Study the drawing (mm; zero at the part's minimum x, y, z) and answer. A direction names the side the tool comes from. Coordinates: 2 decimals unless noted, no trailing zeros. Order: outer loops, then holes, each group sorted by start corner. A loop starts at its lowest first (then second) coordinate and runs counter-clockwise, first axis right, second up. Notation, with made-up numbers: M 27.5,-13.75 L 81.5,-13.75 A16 cw 81.5,6.25 Z; hole C 13,-0.5 d10. An arc over 180 degrees is marked long. Use a Markdown table: item, result. Add a question column.
1) Find section C-C on z = 7.5. Write down the section's boundary in (x, y).
2) Find section D-D on y = 3.25. Write down the section's boundary in (x, z).
3) For the marked faces 1, 2 and 3, determine the directions among +Z, -Z, +X, -X, +Y, -Y from which every point of the face is accessible in a straight line to the end or side of a thin tool.
4) Each of these flat-tipped pins is pushed along its axis until it touches: pin 1 Ø1.5 at (y, z) = (15, 16) entering from +X; pin 2 Ø1 at (x, z) = (5.5, 5) entering from -Y; pin 3 Ø3 at (x, z) = (5, 15.5) entering from -Y; pin 4 Ø1 at (x, z) = (3, 9.5) entering from +Y. Where does it stop, or does it pass through?
5) Find section A-A on y = 10.16. Write down the section's boundary in (x, z), plus the area to 3 significant figures.
6) Find the intervals of material crossed by probe 1 along Z at (x, y) = (17.25, 16.25); probe 2 along Y at (x, z) = (5, 22); probe 3 along Y at (x, z) = (8.75, 7.5), in increasing order. Write a range as [from, to].
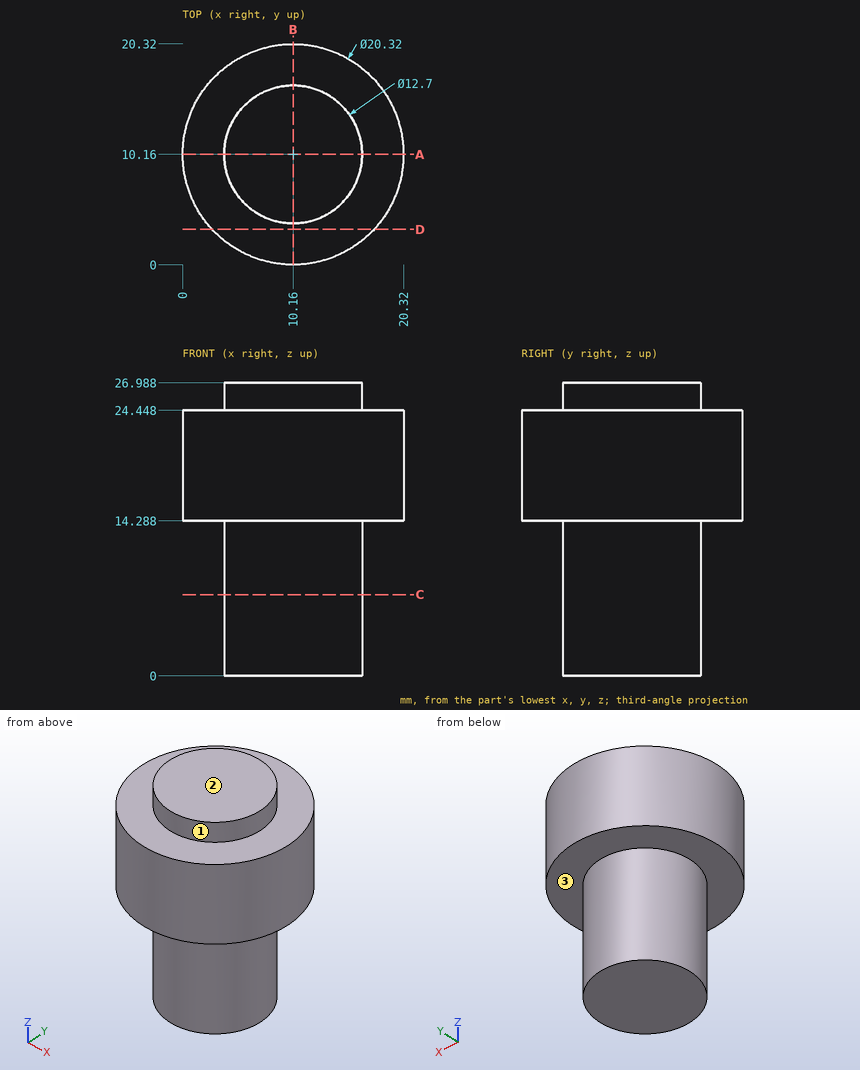
Check result:
| question | item | result |
|---|---|---|
| 1 | outline | C 10.16,10.16 d12.7 |
| 2 | outline | M 2.71,14.29 L 17.61,14.29 L 17.61,24.45 L 2.71,24.45 Z |
| 3 | face 1 | +Z |
| 3 | face 2 | +Z, +X, -X, +Y, -Y |
| 3 | face 3 | -Z |
| 4 | pin 1 | stops at x = 19.46 |
| 4 | pin 2 | stops at y = 5.36 |
| 4 | pin 3 | stops at y = 0.68 |
| 4 | pin 4 | passes through |
| 5 | outline | M 0,14.29 L 3.81,14.29 L 3.81,0 L 16.51,0 L 16.51,14.29 L 20.32,14.29 L 20.32,24.45 L 16.51,24.45 L 16.51,26.99 L 3.81,26.99 L 3.81,24.45 L 0,24.45 Z |
| 5 | area | 420 mm2 |
| 6 | probe 1 | z = [14.29, 24.45] |
| 6 | probe 2 | y = [1.41, 18.91] |
| 6 | probe 3 | y = [3.97, 16.35] |
